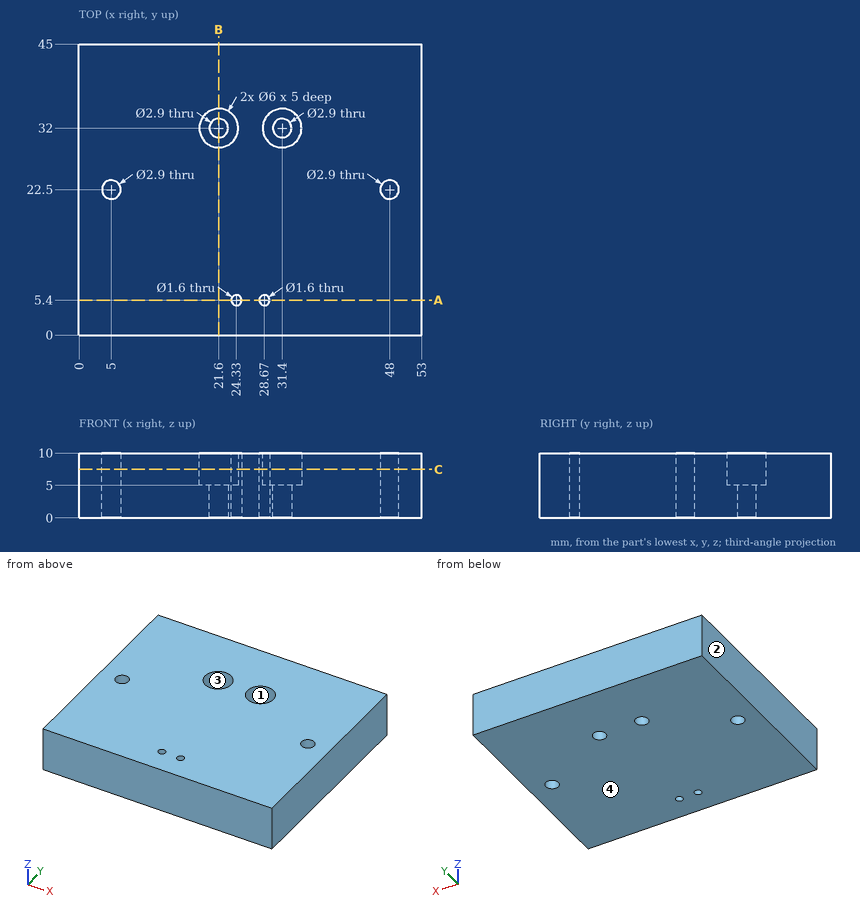
Could you check a few things on this drawing? It's one solid part, dimensions in mm from its lowest x, y, z. Round coordinates to 2 decimals unless told otherwise and drop trailing zeros. Write each loop counter-clockwise with the first axis right and the second up, starting at its lowest first coordinate (ties: lowest second). Pieces come first, ordered by that corner, then holes.
Q1. If we section it at C-C on z = 7.5: Write out the boundary of the cut face in (x, y).
Q2. Please list where these lines run through material, in increasing order: probe 1 along Y at (x, z) = (5, 3.75); probe 2 along Y at (x, z) = (24.33, 4.25); probe 3 along X at (y, z) = (21.5, 3.25).
Q3. If we section it at B-B on x = 21.6: Write out the boundary of the cut face in (y, z).
Q4. Will this pin go through, and if not, where does the flat tip stop? P1, Ø3.5, axis at x = 31.4, y = 32, coming from the +Z side.
Q5. If we section it at A-A on y = 5.4: Write out the boundary of the cut face in (x, z), plus the area to 3 significant figures.
Q6. If we mould it in two halves opening along X, with no side actions, what happens to the marked faces 1, 2, 3 and 4? For each: +X half, -X half, draft (parallel to the pull), parting line (faces both ways), or undercut.
Answer below:
1. outline: (0, 0) - (53, 0) - (53, 45) - (0, 45) - close; hole circle Ø2.9 at (5, 22.5); hole circle Ø6 at (21.6, 32); hole circle Ø1.6 at (24.33, 5.4); hole circle Ø1.6 at (28.67, 5.4); hole circle Ø6 at (31.4, 32); hole circle Ø2.9 at (48, 22.5)
2. probe 1: y = 0 to 21.05, 23.95 to 45
2. probe 2: y = 0 to 4.6, 6.2 to 45
2. probe 3: x = 0 to 3.95, 6.05 to 46.95, 49.05 to 53
3. outline: (0, 0) - (30.55, 0) - (30.55, 5) - (29, 5) - (29, 10) - (0, 10) - close; (33.45, 0) - (45, 0) - (45, 10) - (35, 10) - (35, 5) - (33.45, 5) - close
4. P1: stops at z = 5
5. outline: (0, 0) - (23.53, 0) - (23.53, 10) - (0, 10) - close; (25.13, 0) - (27.87, 0) - (27.87, 10) - (25.13, 10) - close; (29.47, 0) - (53, 0) - (53, 10) - (29.47, 10) - close
5. area: 498 mm2
6. face 1: undercut
6. face 2: -X half
6. face 3: undercut
6. face 4: draft
